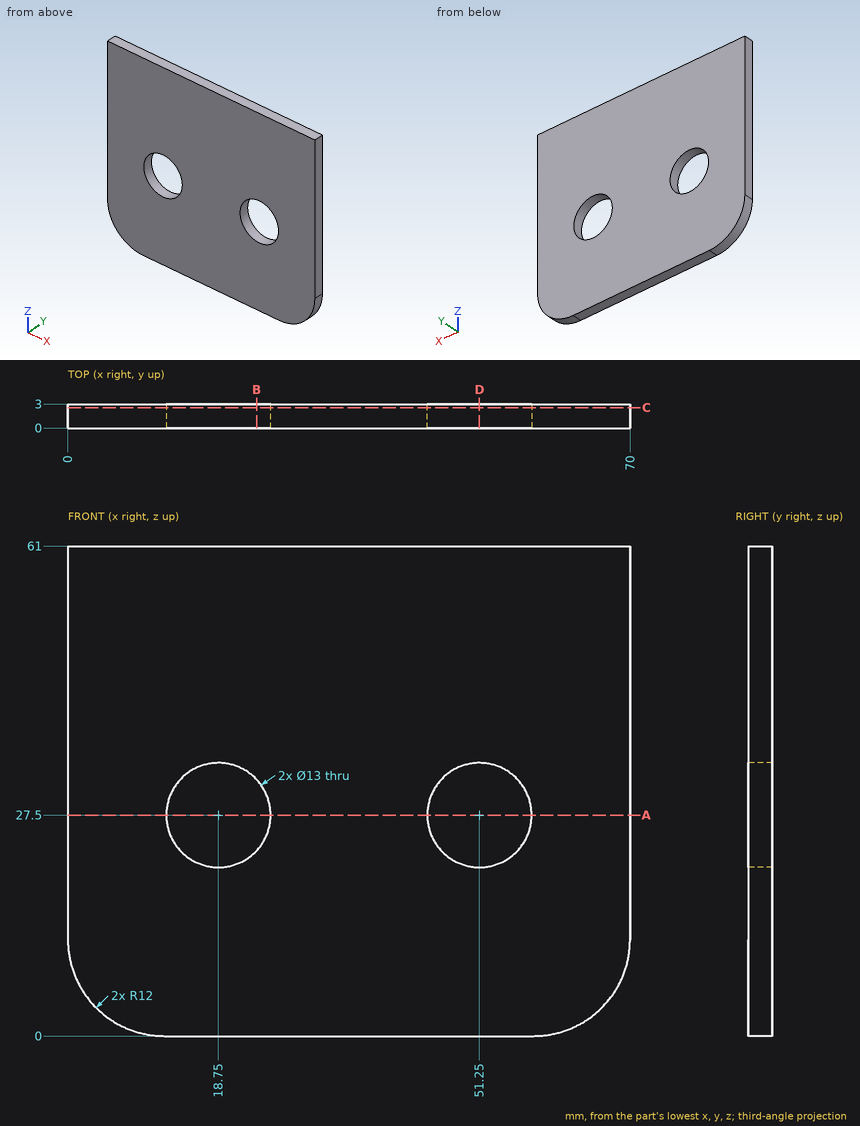
Answer from the drawing. Dimensions are ordinates in mm from the lowest x, y and z of the part. Give positions to 0.01 mm unless a question says otherwise; leave off trailing zeros. Order: outer loops, then holes, each group sorted by start corner. A loop starts at its lowest first (then second) coordinate and runs counter-clockwise, first axis right, second up. Notation, with made-up numbers: (-8.5, -31) - (50.5, -31) arc R25 ccw to (50.5, 4) - close; hole circle Ø1 at (-24.75, 24). An arc over 180 degrees is marked (long way). One line per item, written item: value. Start each with the question number.
1) Given pin 1 Ø1 at (x, y) = (61, 1.5) entering from -Z; pin 2 Ø15 at (x, z) = (51.25, 27.5) entering from -Y; pin 3 Ø11.5 at (x, z) = (18.75, 27.5) entering from +Y, each flat-ended and moving along its own axis, determine where each tip first touches the part or whether it passes through.
2) Find the intervals of material crossed by L1, parallel to Z at x = 18.75, y = 2.4; L2, parallel to X at y = 0.3, z = 25.5; L3, parallel to Z at x = 57, y = 1.85, in increasing order.
3) A cutting plane is placed at D-D on x = 51.25. Give the vertices of the cut face in (y, z), then the cut area to 3 significant figures.
4) A cutting plane is placed at A-A on z = 27.5. Give the vertices of the cut face in (x, y), then the cut area to 3 significant figures.
5) A cutting plane is placed at B-B on x = 23.5. Give the vertices of the cut face in (y, z), then the cut area to 3 significant figures.
6) A cutting plane is placed at C-C on y = 2.55. Give the vertices of the cut face in (x, z).
Answer sheet:
1. pin 1: stops at z = 0.26
1. pin 2: stops at y = 0
1. pin 3: passes through
2. L1: z = 0 to 21, 34 to 61
2. L2: x = 0 to 12.57, 24.93 to 45.07, 57.43 to 70
2. L3: z = 0 to 24.47, 30.53 to 61
3. outline: (0, 0) - (3, 0) - (3, 21) - (0, 21) - close; (0, 34) - (3, 34) - (3, 61) - (0, 61) - close
3. area: 144 mm2
4. outline: (0, 0) - (12.25, 0) - (12.25, 3) - (0, 3) - close; (25.25, 0) - (44.75, 0) - (44.75, 3) - (25.25, 3) - close; (57.75, 0) - (70, 0) - (70, 3) - (57.75, 3) - close
4. area: 132 mm2
5. outline: (0, 0) - (3, 0) - (3, 23.06) - (0, 23.06) - close; (0, 31.94) - (3, 31.94) - (3, 61) - (0, 61) - close
5. area: 156 mm2
6. outline: (0, 12) arc R12 ccw to (12, 0) - (58, 0) arc R12 ccw to (70, 12) - (70, 61) - (0, 61) - close; hole circle Ø13 at (18.75, 27.5); hole circle Ø13 at (51.25, 27.5)
